Answer from the drawing. Dimensions are ordinates in mm from the lowest x, y and z of the part. A direction names the side the tool comes from. Coordinates: 2 decimals unless noted, no trailing zeros. Order: outer loops, then holes, each group sorted by start corner. A loop starts at its lowest first (then second) coordinate and runs counter-clockwise, first axis right, second up. Notation, with made-up numbers: M 70,10.5 L 108,10.5 A12 cw 108,28.5 Z; hole C 89.25,-26.5 d2. An arc over 180 degrees is marked long. Use a Markdown table: item, result.
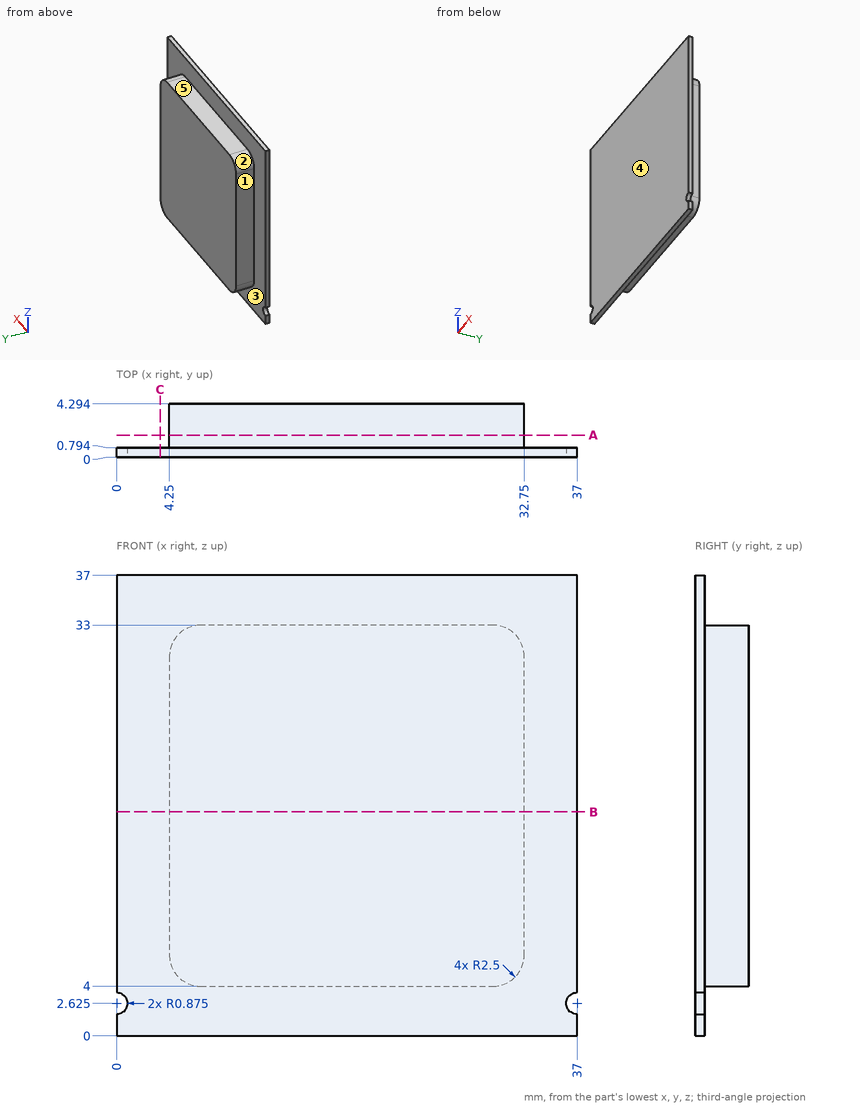
(1) A cutting plane is placed at B-B (z = 18). Determine the outline of the cut face in (x, y).
Conclusion:
| item | result |
|---|---|
| outline | M 0,0 L 37,0 L 37,0.79 L 32.75,0.79 L 32.75,4.29 L 4.25,4.29 L 4.25,0.79 L 0,0.79 Z |
(2) A cutting plane is placed at A-A (y = 1.8). Determine the outline of the cut face in (x, z).
Conclusion:
| item | result |
|---|---|
| outline | M 4.25,6.5 A2.5 ccw 6.75,4 L 30.25,4 A2.5 ccw 32.75,6.5 L 32.75,30.5 A2.5 ccw 30.25,33 L 6.75,33 A2.5 ccw 4.25,30.5 Z |
(3) Given P1, Ø1.8, axis at x = 13, y = 2, coming from the -Z side; P2, Ø1.5, axis at y = 3.5, z = 10, coming from the +X side; P3, Ø1.8, axis at x = 16, y = 3.5, coming from the +Z side, each flat-ended and moving along its own axis, determine where each tip first touches the part or whether it passes through.
Conclusion:
| item | result |
|---|---|
| P1 | z = 4 |
| P2 | x = 32.75 |
| P3 | z = 33 |
(4) Straight lines are drawn through the part: L1, parallel to X at y = 2.3, z = 15.5; L2, parallel to Z at x = 12.5, y = 3; L3, parallel to Y at x = 27, z = 33.5. For each, find the intervals that lie inside material, in ascending order.
Conclusion:
| item | result |
|---|---|
| L1 | 4.25 to 32.75 |
| L2 | 4 to 33 |
| L3 | 0 to 0.79 |
(5) Which of the six approach directions +Z, -Z, +X, -X, +Y, -Y give full straight-line access (tool end or side, diameter ignored) to the marked faces 1, 2, 3, 4 and 5?
Conclusion:
| item | result |
|---|---|
| face 1 | +Z, -Z, -X, +Y |
| face 2 | +Z, -X, +Y |
| face 3 | +Y |
| face 4 | +Z, -Z, +X, -X, -Y |
| face 5 | +Z, +X, -X, +Y |
(6) A cutting plane is placed at C-C (x = 3.5). Determine the outline of the cut face in (y, z).
Conclusion:
| item | result |
|---|---|
| outline | M 0,0 L 0.79,0 L 0.79,37 L 0,37 Z |
